Model file for the job. Use its own axes, mm. A direction names the side the tool comes from. Round coordinates to 2 decimals unless told otherwise and drop trailing zeros. Order: outer loops, then holes, each group sorted by start corner. A loop starts at its lowest first (then second) coordinate and runs counter-clockwise, first axis right, second up. Notation, with made-up numbers: (80.5, 28.5) -> (139.5, 28.5) arc R8 ccw to (139.5, 37.5) -> close; hole circle Ø8 at (2, 41). An arc over 180 degrees is marked (long way). Put each result on its own line as item: value. Start each with the question number.
Q1. Probe L1, parallel to X at y = 3.95, z = -2; L2, parallel to X at y = 0.85, z = 4; L3, parallel to Z at x = 14.25, y = 1. List the from-to ranges inside material, lowest first.
Q2. Flat gauge pins, fed straight in: P1, Ø5.5, axis at x = 5.5, z = 3, coming from the +Y side; P2, Ø8, axis at x = 9, y = 3, coming from the -Z side; P3, Ø2, axis at x = 14, y = 8, coming from the +Z side; P4, Ø1, axis at x = 8.5, y = 0.5, coming from the -Z side. Where does each tip first touch, or does it go through?
Q3. Cut at A-A, the plane y = 3.95. List the corners of the cut face in (x, z), and give its area (3 significant figures).
Q4. Cut at C-C, the plane y = 11.95. List the corners of the cut face in (x, z).
Q5. 3-axis set-ups, long thin cutter, end or side, ignore diameter. For faces 1 (the face through (13, 4, -1.584)), 2 (the face through (9, 0, 7)), 3 (the face through (8, 1, 6.7)): which of +Z, -Z, +X, -X, +Y, -Y reach the whole face in a straight line?
Q6. Pull direction Z, two halves, no side cores. Call faces 4 (the face through (4.148, 9.998, -2.496)), 5 (the face through (10.184, 3.989, 3.894)), 6 (the face through (5, 4, -1.584)): released by +Z, released by -Z, zero draft, split by the parting line, or undercut.
from build123d import *

# Parameters (mm, degrees)
MAINBASESKETCH_W                       = 15.8
MAINBASESKETCH_H                       = 3.2
MAINBASEEXTRUDE_DEPTH                  = 7.9
STUDSSKETCH_R                          = 2.4
STUDSEXTRUDE_DEPTH                     = 1.6
STUDSPATTERN_COUNT                     = 2
STUDSPATTERN_PITCH                     = 8
STUDSPATTERN_COUNT_DIR2                = 2
STUDSPATTERN_PITCH_DIR2                = 8
MAINBASESHELL_T                        = -1.2
LCUTBLUE_DEPTH                         = 19.555463972
LCUTBLUE_DEPTH_BACK                    = 19.555463972
CUTADDEDTOLCUT_DEPTH                   = 2
MADESLIMCUTSKETCH_W                    = 7.9
MADESLIMCUTSKETCH_H                    = 7.9
MADESLIMCUT_DEPTH                      = 19.897228453
MADESLIMFILLEXT_REACH                  = 20.897
SKETCH33_W                             = 5.500952983
SKETCH33_H                             = 1.199047018
SLIMHOLEEXT_START                      = -0.2
SLIMHOLESKETCH_R                       = 1.75
SLIMHOLESKETCH_R_2                     = 0.75
SLIMHOLEEXT_DEPTH                      = 2
SHORTLEXTENSIONSKETCH_W                = 1.583745828
SHORTLEXTENSIONSKETCH_H                = 7.9
SHORTLEXTENDEDCUTSKETCH_W              = 13.4
SHORTLEXTENDEDCUTSKETCH_H              = 1.582792846
SHORTLEXTENDEDCUT_DEPTH                = 2
SHORTLUNDERSTUMPS_START                = -0.2
SHORTLUNDERSTUMPSKETCH_W               = 0.996828098
SHORTLUNDERSTUMPSKETCH_H               = 1.1
SHORTLUNDERSTUMPS_DEPTH                = 1.5
SHORTLUPPERCIRCLES_START               = -0.2
SHORTLUPPERCIRCLESSKETCH_R             = 2.4
SHORTLUPPERCIRCLESSKETCH_R_2           = 2
SHORTLUPPERCIRCLESSKETCH_R_3           = 2.45
SHORTLUPPERCIRCLES_DEPTH               = 2
TALLERLBASEEXTENSIONSKETCH_W           = 1.583745828
TALLERLBASEEXTENSIONSKETCH_H           = 7.48
F_4UPPERCIRCLESTALLERLBASE_START       = -3.383745828
F_4UPPERCIRCLESTALLERLBASE_OUTLINE_R   = 2.45
F_4UPPERCIRCLESTALLERLBASE_OUTLINE_R_2 = 2
F_4UPPERCIRCLESTALLERLBASE_OUTLINE_R_3 = 2.4
F_4UPPERCIRCLESTALLERLBASE_DEPTH       = 1.8
TALLERLBASEOUTERCHAMFER_R              = 1


# Read off the part's stored shape, not the designer's step: 4UpperCirclesTallerLBase
with BuildPart() as part:
    # MainBaseSketch → MainBaseExtrude (new, symmetric)
    with BuildSketch(Plane.XY):
        with Locations((8.581967213, 1.6)):
            Rectangle(MAINBASESKETCH_W, MAINBASESKETCH_H)
    extrude(amount=MAINBASEEXTRUDE_DEPTH, both=True)

    # StudsSketch → StudsExtrude (add)
    with BuildSketch(Plane(origin=(0, 3.2, 0), x_dir=(1, 0, 0), z_dir=(0, 1, 0))):
        with Locations((4.581967213, 4)):
            Circle(STUDSSKETCH_R)
    studsextrude = extrude(amount=STUDSEXTRUDE_DEPTH)

    # StudsPattern: StudsExtrude 2 × 2
    with Locations(*[(j * STUDSPATTERN_PITCH_DIR2, 0, i * STUDSPATTERN_PITCH) for i in range(STUDSPATTERN_COUNT) for j in range(STUDSPATTERN_COUNT_DIR2) if (i, j) != (0, 0)]):
        add(studsextrude)

    # MainBaseShell
    mainbaseshell_openings = [part.faces().sort_by_distance(p)[0] for p in [
        (8.581967213, 0, 0),
    ]]
    offset(amount=MAINBASESHELL_T, openings=mainbaseshell_openings, kind=Kind.INTERSECTION)

    # LCUTBlueSketch → LCutBlue (cut, two sides: drawn at the far end of the back side and taken through both)
    with BuildSketch(Plane(origin=(0, 3.2, 0), x_dir=(1, 0, 0), z_dir=(0, 1, 0)).offset(-LCUTBLUE_DEPTH_BACK)):
        Polygon((8.581967213, 53.229874044), (8.581967213, 7.9), (8.581967213, 0), (16.481967213, 0), (61.811841258, 0), (125.917963912, 64.106122654), (72.688089868, 117.335996699), align=None)
    extrude(amount=LCUTBLUE_DEPTH + LCUTBLUE_DEPTH_BACK, mode=Mode.SUBTRACT)

    # CutAddedtoLSketch → CutAddedToLCut (add)
    with BuildSketch(Plane.XZ):
        Polygon((7.382920196, -6.7), (8.581967213, -6.7), (8.581967213, 0), (15.281967213, 0), (15.281967213, 1.199047018), (7.382920196, 1.199047018), (7.382920196, 0), align=None)
    extrude(amount=-CUTADDEDTOLCUT_DEPTH)

    # MadeSlimCutSketch → MadeSlimCut (cut, through all)
    with BuildSketch(Plane.XZ):
        with Locations((4.631967213, -3.95)):
            Rectangle(MADESLIMCUTSKETCH_W, MADESLIMCUTSKETCH_H)
    extrude(amount=-MADESLIMCUT_DEPTH, mode=Mode.SUBTRACT)

    # Sketch33 → MadeSlimFillExt (add, up to next)
    with BuildSketch(Plane.XZ, mode=Mode.PRIVATE) as madeslimfillext_sk1:
        with Locations((4.632443704, 0.599523509)):
            Rectangle(SKETCH33_W, SKETCH33_H)
    madeslimfillext_tool1 = extrude(madeslimfillext_sk1.sketch, amount=-MADESLIMFILLEXT_REACH, mode=Mode.PRIVATE) - part.part
    add(madeslimfillext_tool1.solids().sort_by_distance((4.632444, 0, 0.599524))[0])

    # SlimHoleSketch → SlimHoleExt (add)
    with BuildSketch(Plane.XZ.offset(-2).offset(SLIMHOLEEXT_START)):
        with Locations((8.581967213, 4)):
            Circle(SLIMHOLESKETCH_R)
        with Locations((8.581967213, 4)):
            Circle(SLIMHOLESKETCH_R_2, mode=Mode.SUBTRACT)
    extrude(amount=SLIMHOLEEXT_DEPTH)

    # ShortLExtension: sweep along a curve in space
    with BuildLine() as shortlextension_path:
        Line((0.681967213, 3.2, 0), (16.481967213, 3.2, 0))
    # ShortLExtensionSketch → ShortLExtension (sweep)
    with BuildSketch(Plane(origin=(16.481967213, 0, 0), x_dir=(0, 0, -1), z_dir=(1, 0, 0))):
        with Locations((0.791872914, 3.95)):
            Rectangle(SHORTLEXTENSIONSKETCH_W, SHORTLEXTENSIONSKETCH_H)
    sweep(path=shortlextension_path.line)

    # ShortLExtendedCutSketch → ShortLExtendedCut (cut)
    with BuildSketch(Plane.XZ):
        with Locations((8.581967213, 0.407650595)):
            Rectangle(SHORTLEXTENDEDCUTSKETCH_W, SHORTLEXTENDEDCUTSKETCH_H)
    extrude(amount=-SHORTLEXTENDEDCUT_DEPTH, mode=Mode.SUBTRACT)

    # ShortLUnderStumpSketch → ShortLUnderStumps (add)
    with BuildSketch(Plane.XZ.offset(-2).offset(SHORTLUNDERSTUMPS_START)):
        with Locations((4.581764801, 0.166254172)):
            Rectangle(SHORTLUNDERSTUMPSKETCH_W, SHORTLUNDERSTUMPSKETCH_H)
        with Locations((8.57767054, 0.166254172)):
            Rectangle(SHORTLUNDERSTUMPSKETCH_W, SHORTLUNDERSTUMPSKETCH_H)
        with Locations((12.582169625, 0.166254172)):
            Rectangle(SHORTLUNDERSTUMPSKETCH_W, SHORTLUNDERSTUMPSKETCH_H)
    extrude(amount=SHORTLUNDERSTUMPS_DEPTH)

    # ShortLUpperCirclesSketch → ShortLUpperCircles (add)
    # profile 1 of 2: a face of its own
    with BuildSketch(Plane(origin=(0, 0, -1.583745828), x_dir=(-1, 0, 0), z_dir=(0, 0, -1)).offset(SHORTLUPPERCIRCLES_START)):
        with Locations(Location((-12.581967213, 3.95, 0), (0, 0, 90))):
            Circle(SHORTLUPPERCIRCLESSKETCH_R)
        with Locations(Location((-12.581967213, 3.95, 0), (0, 0, 90))):
            Circle(SHORTLUPPERCIRCLESSKETCH_R_2, mode=Mode.SUBTRACT)
    # profile 2 of 2: a face of its own
    with BuildSketch(Plane(origin=(0, 0, -1.583745828), x_dir=(-1, 0, 0), z_dir=(0, 0, -1)).offset(SHORTLUPPERCIRCLES_START)):
        with Locations(Location((-4.581967213, 3.95, 0), (0, 0, 270))):
            Circle(SHORTLUPPERCIRCLESSKETCH_R_3)
        with Locations(Location((-4.581967213, 3.95, 0), (0, 0, 270))):
            Circle(SHORTLUPPERCIRCLESSKETCH_R_2, mode=Mode.SUBTRACT)
    extrude(amount=SHORTLUPPERCIRCLES_DEPTH)

    # TallerLBaseExtension: sweep along a curve in space
    with BuildLine() as tallerlbaseextension_path:
        Line((0.681967213, 7.9, -1.583745828), (16.481967213, 7.9, -1.583745828))
    # TallerLBaseExtensionSketch → TallerLBaseExtension (sweep)
    with BuildSketch(Plane(origin=(16.481967213, 0, 0), x_dir=(0, 0, -1), z_dir=(1, 0, 0))):
        with Locations((0.791872914, 11.64)):
            Rectangle(TALLERLBASEEXTENSIONSKETCH_W, TALLERLBASEEXTENSIONSKETCH_H)
    sweep(path=tallerlbaseextension_path.line)

    # 4UpperCirclesTallerLBase outline → 4UpperCirclesTallerLBase (add)
    # profile 1 of 2: a face of its own
    with BuildSketch(Plane.XY.offset(F_4UPPERCIRCLESTALLERLBASE_START)):
        with Locations((4.581967213, 11.95)):
            Circle(F_4UPPERCIRCLESTALLERLBASE_OUTLINE_R)
        with Locations((4.581967213, 11.95)):
            Circle(F_4UPPERCIRCLESTALLERLBASE_OUTLINE_R_2, mode=Mode.SUBTRACT)
    # profile 2 of 2: a face of its own
    with BuildSketch(Plane.XY.offset(F_4UPPERCIRCLESTALLERLBASE_START)):
        with Locations((12.581967213, 11.95)):
            Circle(F_4UPPERCIRCLESTALLERLBASE_OUTLINE_R_3)
        with Locations((12.581967213, 11.95)):
            Circle(F_4UPPERCIRCLESTALLERLBASE_OUTLINE_R_2, mode=Mode.SUBTRACT)
    extrude(amount=F_4UPPERCIRCLESTALLERLBASE_DEPTH)

    # TallerLBaseOuterChamfer
    tallerlbaseouterchamfer_edges = [part.edges().sort_by_distance(p)[0] for p in [
        (16.481967213, 15.38, -0.791872914),
        (0.681967213, 15.38, -0.791872914),
    ]]
    fillet(tallerlbaseouterchamfer_edges, radius=TALLERLBASEOUTERCHAMFER_R)


solid = part.part
Ans:
1. L1: x = 2.13 to 2.58, 6.58 to 7.03, 10.18 to 10.58, 14.58 to 14.98
1. L2: x = 0.68 to 1.88, 6.83 to 7.83, 9.33 to 10.33, 15.28 to 16.48
1. L3: z = -1.58 to -0.38, 6.7 to 7.9
2. P1: stops at y = 4.8
2. P2: stops at z = -3.38
2. P3: stops at z = 0
2. P4: stops at z = -1.58
3. outline: (0.68, -1.58) -> (2.13, -1.58) -> (2.13, -3.38) -> (2.58, -3.38) -> (2.58, -1.58) -> (6.58, -1.58) -> (6.58, -3.38) -> (7.03, -3.38) -> (7.03, -1.58) -> (10.18, -1.58) -> (10.18, -3.38) -> (10.58, -3.38) -> (10.58, -1.58) -> (14.58, -1.58) -> (14.58, -3.38) -> (14.98, -3.38) -> (14.98, -1.58) -> (16.48, -1.58) -> (16.48, 0) -> (0.68, 0) -> close; circle Ø4.8 at (4.58, 4); circle Ø4.8 at (12.58, 4)
3. area: 64.3 mm^2
4. outline: (0.68, -1.58) -> (2.13, -1.58) -> (2.13, -3.38) -> (2.58, -3.38) -> (2.58, -1.58) -> (6.58, -1.58) -> (6.58, -3.38) -> (7.03, -3.38) -> (7.03, -1.58) -> (10.18, -1.58) -> (10.18, -3.38) -> (10.58, -3.38) -> (10.58, -1.58) -> (14.58, -1.58) -> (14.58, -3.38) -> (14.98, -3.38) -> (14.98, -1.58) -> (16.48, -1.58) -> (16.48, 0) -> (0.68, 0) -> close
5. face 1: -Z
5. face 2: +Z, -Z, +X, -X, -Y
5. face 3: -Y
6. face 4: zero draft
6. face 5: undercut
6. face 6: released by -Z
